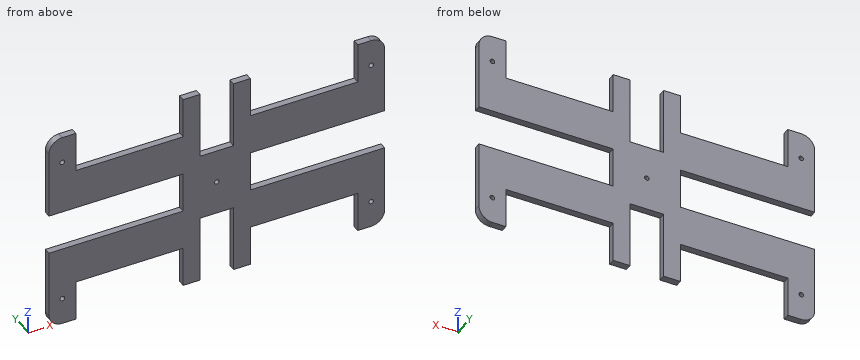
from build123d import *

# Parameters (mm, degrees)
SKETCH_1_W                                 = 250
SKETCH_1_H                                 = 150
EXTRUDE_1_DEPTH                            = 5
FILLET_1_R                                 = 10
SKETCH_2_R                                 = 1.75
CUT_EXTRUDE_1_DEPTH                        = 146.859521458
MIRROR_2_COPY_1_SKETCH_R                   = 1.75
MIRROR_2_COPY_1_DEPTH                      = 146.859521458
SKETCH_4_R                                 = 1.75
CUT_EXTRUDE_2_DEPTH                        = 5
SKETCH_5_W                                 = 25
SKETCH_5_H                                 = 50
CUT_EXTRUDE_3_DEPTH                        = 5
SKETCH_7_W                                 = 210
SKETCH_7_H                                 = 30
CUT_EXTRUDE_4_DEPTH                        = 5
SKETCH_8_W                                 = 12.5
SKETCH_8_H                                 = 30
EXTRUDE_2_DEPTH                            = 5
MIRROR_5_AT_THE_SECOND_PLANE_COPY_1_SKET_W = 12.5
MIRROR_5_AT_THE_SECOND_PLANE_COPY_1_SKET_H = 30
MIRROR_5_AT_THE_SECOND_PLANE_COPY_1_DEPTH  = 5
SKETCH_9_W                                 = 100
SKETCH_9_H                                 = 30
CUT_EXTRUDE_5_DEPTH                        = 5


with BuildPart() as part:
    # 草图1 → 凸台-拉伸1 (new body)
    with BuildSketch(Plane(origin=(0, 0, 0), x_dir=(1, 0, 0), z_dir=(0, 1, 0))):
        Rectangle(SKETCH_1_W, SKETCH_1_H)
    extrude(amount=EXTRUDE_1_DEPTH)

    # 圆角1
    fillet_1_edges = [part.edges().sort_by_distance(p)[0] for p in [
        (-125, 2.5, -75),
        (125, 2.5, -75),
        (125, 2.5, 75),
        (-125, 2.5, 75),
    ]]
    fillet(fillet_1_edges, radius=FILLET_1_R)

    # 草图2 → 切除-拉伸1 (cut, symmetric)
    with BuildSketch(Plane(origin=(0, 5, 0), x_dir=(1, 0, 0), z_dir=(0, 1, 0))):
        with Locations(Location((-115, -55, 0), (0, 0, 270))):
            Circle(SKETCH_2_R)
    cut_extrude_1 = extrude(amount=CUT_EXTRUDE_1_DEPTH, both=True, mode=Mode.SUBTRACT)

    # 镜向1: 切除-拉伸1 across plane
    add(cut_extrude_1.mirror(Plane.XY), mode=Mode.SUBTRACT)

    # 镜向2: 切除-拉伸1 across plane
    add(cut_extrude_1.mirror(Plane(origin=(0, 0, 0), x_dir=(0, 0, 1), z_dir=(1, 0, 0))), mode=Mode.SUBTRACT)

    # 镜向2 copy 1 sketch → 镜向2 copy 1 (cut, symmetric)
    with BuildSketch(Plane(origin=(0, 5, 0), x_dir=(-1, 0, 0), z_dir=(0, 1, 0))):
        with Locations(Location((-115, -55, 0), (0, 0, 270))):
            Circle(MIRROR_2_COPY_1_SKETCH_R)
    extrude(amount=MIRROR_2_COPY_1_DEPTH, both=True, mode=Mode.SUBTRACT)

    # 草图4 → 切除-拉伸2 (cut)
    with BuildSketch(Plane(origin=(0, 5, 0), x_dir=(1, 0, 0), z_dir=(0, 1, 0))):
        with Locations(Location((0, 0, 0), (0, 0, 270))):
            Circle(SKETCH_4_R)
    extrude(amount=-CUT_EXTRUDE_2_DEPTH, mode=Mode.SUBTRACT)

    # 草图5 → 切除-拉伸3 (cut)
    with BuildSketch(Plane.XZ):
        with Locations((0, 50)):
            Rectangle(SKETCH_5_W, SKETCH_5_H)
    cut_extrude_3 = extrude(amount=-CUT_EXTRUDE_3_DEPTH, mode=Mode.SUBTRACT)

    # 草图7 → 切除-拉伸4 (cut)
    with BuildSketch(Plane.XZ):
        with Locations((0, -60)):
            Rectangle(SKETCH_7_W, SKETCH_7_H)
    cut_extrude_4 = extrude(amount=-CUT_EXTRUDE_4_DEPTH, mode=Mode.SUBTRACT)

    # 镜向3: 切除-拉伸4 across plane
    add(cut_extrude_4.mirror(Plane.XY), mode=Mode.SUBTRACT)

    # 镜向4: 切除-拉伸3 across plane
    add(cut_extrude_3.mirror(Plane.XY), mode=Mode.SUBTRACT)

    # 草图8 → 凸台-拉伸2 (add)
    with BuildSketch(Plane(origin=(0, 5, 0), x_dir=(1, 0, 0), z_dir=(0, 1, 0))):
        with Locations((-18.75, -60)):
            Rectangle(SKETCH_8_W, SKETCH_8_H)
    extrude_2 = extrude(amount=-EXTRUDE_2_DEPTH)

    # 镜向5: 凸台-拉伸2 across plane
    add(extrude_2.mirror(Plane(origin=(0, 0, 0), x_dir=(0, 0, 1), z_dir=(1, 0, 0))))

    # 镜向5 at the second plane: 凸台-拉伸2 across plane
    add(extrude_2.mirror(Plane.XY))

    # 镜向5 at the second plane copy 1 sket → 镜向5 at the second plane copy 1 (add)
    with BuildSketch(Plane(origin=(0, 5, 0), x_dir=(-1, 0, 0), z_dir=(0, 1, 0))):
        with Locations((-18.75, -60)):
            Rectangle(MIRROR_5_AT_THE_SECOND_PLANE_COPY_1_SKET_W, MIRROR_5_AT_THE_SECOND_PLANE_COPY_1_SKET_H)
    extrude(amount=-MIRROR_5_AT_THE_SECOND_PLANE_COPY_1_DEPTH)

    # 草图9 → 切除-拉伸5 (cut)
    with BuildSketch(Plane(origin=(0, 5, 0), x_dir=(1, 0, 0), z_dir=(0, 1, 0))):
        with Locations((-75, 0)):
            Rectangle(SKETCH_9_W, SKETCH_9_H)
    cut_extrude_5 = extrude(amount=-CUT_EXTRUDE_5_DEPTH, mode=Mode.SUBTRACT)

    # 镜向6: 切除-拉伸5 across plane
    add(cut_extrude_5.mirror(Plane(origin=(0, 0, 0), x_dir=(0, 0, 1), z_dir=(1, 0, 0))), mode=Mode.SUBTRACT)


solid = part.part
For this review, take the finished solid that the model builds, in its own axes (mm). Round coordinates to 2 decimals unless told otherwise and drop trailing zeros. Write each loop counter-clockwise with the first axis right and the second up, starting at its lowest first coordinate (ties: lowest second). Pieces come first, ordered by that corner, then holes. Notation, with made-up numbers: (72.25, -40) -> (118.25, -40) arc R14 ccw to (118.25, -28) -> close; hole circle Ø1 at (28.5, -18). An arc over 180 degrees is marked (long way). Put each result on its own line as item: value.
Q1. Consider section A-A on z = 41. State the section outline as (x, y) points, and give its area (4 significant figures).
Determined:
outline: (-125, 0) -> (-12.5, 0) -> (-12.5, 5) -> (-125, 5) -> close; (12.5, 0) -> (125, 0) -> (125, 5) -> (12.5, 5) -> close
area: 1,125 mm^2
Q2. To check wall thickness, follow L1, parallel to Z at x = 115, y = 1.45; L2, parallel to X at y = 3.4, z = 55; L3, parallel to X at y = 4.2, z = 59.5. State the ranges of each line that lie inside material, in increasing order. Write a range as [from, to].
Determined:
L1: z = [-75, -56.75], [-53.25, -15], [15, 53.25], [56.75, 75]
L2: x = [-125, -116.75], [-113.25, -105], [-25, -12.5], [12.5, 25], [105, 113.25], [116.75, 125]
L3: x = [-125, -105], [-25, -12.5], [12.5, 25], [105, 125]
Q3. Consider section D-D on z = 6.5. State the section outline as (x, y) points, and give its area (3 significant figures).
Determined:
outline: (-25, 0) -> (25, 0) -> (25, 5) -> (-25, 5) -> close
area: 250 mm^2
Q4. Clearance check with flat-ended pins moving along their axes: pin 1 Ø1.5 at (x, y) = (47, 4) entering from -Z; pin 2 Ø1.5 at (y, z) = (2, 3.5) entering from +X. State where each tip first meets the part, or that it passes through.
Determined:
pin 1: stops at z = -45
pin 2: stops at x = 25
Q5. Consider section B-B on x = -45. State the section outline as (y, z) points.
Determined:
outline: (0, -45) -> (5, -45) -> (5, -15) -> (0, -15) -> close; (0, 15) -> (5, 15) -> (5, 45) -> (0, 45) -> close
Q6. Consider section C-C on y = 1.9. Give the number of separate pieces and of enclosed holes in the cut face, and give its area (3 significant figures).
Determined:
separate pieces: 1
enclosed holes: 5
area: 19,300 mm^2
